```python
from build123d import *

# Parameters (mm, degrees)
F0_R          = 3
F0_R_2        = 2.5
F1_DEPTH      = 1100.6
F2_R          = 2
F3_R          = 7
F5_DEPTH      = 30
F5_DEPTH_BACK = 30


# Not quite as in the source:
# - a feature names something its author has since deleted; it is built from what else it names


with BuildPart() as f1:
    # F0 (on Top) → F1 (new body)
    with BuildSketch(Plane.XY):
        with BuildLine():
            Line((18.15, -30), (30, -30))
            Line((30, -30), (30, -18.15))
            Line((30, -18.15), (27.5, -18.15))
            Line((27.5, -18.15), (27.5, -20.15))
            Line((27.5, -20.15), (21.5477069044, -20.15))
            ThreePointArc((21.5477069044, -20.15), (19.5, -15), (21.5477069044, -9.85))
            Line((21.5477069044, -9.85), (27.5, -9.85))
            Line((27.5, -9.85), (27.5, -11.85))
            Line((27.5, -11.85), (30, -11.85))
            Line((30, -11.85), (30, 11.85))
            Line((30, 11.85), (27.5, 11.85))
            Line((27.5, 11.85), (27.5, 9.85))
            Line((27.5, 9.85), (21.5477069044, 9.85))
            ThreePointArc((21.5477069044, 9.85), (19.5, 15), (21.5477069044, 20.15))
            Line((21.5477069044, 20.15), (27.5, 20.15))
            Line((27.5, 20.15), (27.5, 18.15))
            Line((27.5, 18.15), (30, 18.15))
            Line((30, 18.15), (30, 30))
            Line((30, 30), (18.15, 30))
            Line((18.15, 30), (18.15, 27.5))
            Line((18.15, 27.5), (20.15, 27.5))
            Line((20.15, 27.5), (20.15, 21.5477069044))
            ThreePointArc((20.15, 21.5477069044), (15, 19.5), (9.85, 21.5477069044))
            Line((9.85, 21.5477069044), (9.85, 27.5))
            Line((9.85, 27.5), (11.85, 27.5))
            Line((11.85, 27.5), (11.85, 30))
            Line((11.85, 30), (-11.85, 30))
            Line((-11.85, 30), (-11.85, 27.5))
            Line((-11.85, 27.5), (-9.85, 27.5))
            Line((-9.85, 27.5), (-9.85, 21.5477069044))
            ThreePointArc((-9.85, 21.5477069044), (-15, 19.5), (-20.15, 21.5477069044))
            Line((-20.15, 21.5477069044), (-20.15, 27.5))
            Line((-20.15, 27.5), (-18.15, 27.5))
            Line((-18.15, 27.5), (-18.15, 30))
            Line((-18.15, 30), (-30, 30))
            Line((-30, 30), (-30, 18.15))
            Line((-30, 18.15), (-27.5, 18.15))
            Line((-27.5, 18.15), (-27.5, 20.15))
            Line((-27.5, 20.15), (-21.5477069044, 20.15))
            ThreePointArc((-21.5477069044, 20.15), (-19.5, 15), (-21.5477069044, 9.85))
            Line((-21.5477069044, 9.85), (-27.5, 9.85))
            Line((-27.5, 9.85), (-27.5, 11.85))
            Line((-27.5, 11.85), (-30, 11.85))
            Line((-30, 11.85), (-30, -11.85))
            Line((-30, -11.85), (-27.5, -11.85))
            Line((-27.5, -11.85), (-27.5, -9.85))
            Line((-27.5, -9.85), (-21.5477069044, -9.85))
            ThreePointArc((-21.5477069044, -9.85), (-19.5, -15), (-21.5477069044, -20.15))
            Line((-21.5477069044, -20.15), (-27.5, -20.15))
            Line((-27.5, -20.15), (-27.5, -18.15))
            Line((-27.5, -18.15), (-30, -18.15))
            Line((-30, -18.15), (-30, -30))
            Line((-30, -30), (-18.15, -30))
            Line((-18.15, -30), (-18.15, -27.5))
            Line((-18.15, -27.5), (-20.15, -27.5))
            Line((-20.15, -27.5), (-20.15, -21.5477069044))
            ThreePointArc((-20.15, -21.5477069044), (-15, -19.5), (-9.85, -21.5477069044))
            Line((-9.85, -21.5477069044), (-9.85, -27.5))
            Line((-9.85, -27.5), (-11.85, -27.5))
            Line((-11.85, -27.5), (-11.85, -30))
            Line((-11.85, -30), (11.85, -30))
            Line((11.85, -30), (11.85, -27.5))
            Line((11.85, -27.5), (9.85, -27.5))
            Line((9.85, -27.5), (9.85, -21.5477069044))
            ThreePointArc((9.85, -21.5477069044), (15, -19.5), (20.15, -21.5477069044))
            Line((20.15, -21.5477069044), (20.15, -27.5))
            Line((20.15, -27.5), (18.15, -27.5))
            Line((18.15, -27.5), (18.15, -30))
        make_face()
        with Locations((-25, -25)):
            Circle(F0_R, mode=Mode.SUBTRACT)
        with Locations((-15, -15)):
            Circle(F0_R_2, mode=Mode.SUBTRACT)
        with Locations((25, -25)):
            Circle(F0_R, mode=Mode.SUBTRACT)
        with Locations((15, -15)):
            Circle(F0_R_2, mode=Mode.SUBTRACT)
        with Locations((-25, 25)):
            Circle(F0_R, mode=Mode.SUBTRACT)
        with Locations((-15, 15)):
            Circle(F0_R_2, mode=Mode.SUBTRACT)
        Polygon((-7, 22), (-7, 27.5), (0, 27.5), (7, 27.5), (7, 22), (10, 16), (10, 10), (16, 10), (22, 7), (27.5, 7), (27.5, 0), (27.5, -7), (22, -7), (16, -10), (10, -10), (10, -16), (7, -22), (7, -27.5), (0, -27.5), (-7, -27.5), (-7, -22), (-10, -16), (-10, -10), (-16, -10), (-22, -7), (-27.5, -7), (-27.5, 0), (-27.5, 7), (-22, 7), (-16, 10), (-10, 10), (-10, 16), align=None, mode=Mode.SUBTRACT)
        with Locations((15, 15)):
            Circle(F0_R_2, mode=Mode.SUBTRACT)
        with Locations((25, 25)):
            Circle(F0_R, mode=Mode.SUBTRACT)
    extrude(amount=F1_DEPTH)

    # F2
    f2_edges = [f1.edges().sort_by_distance(p)[0] for p in [
        (-7, 27.5, 550.3),
        (7, 27.5, 550.3),
    ]]
    fillet(f2_edges, radius=F2_R)

    # F3
    f3_edges = [f1.edges().sort_by_distance(p)[0] for p in [
        (-10, 16, 550.3),
        (10, 16, 550.3),
    ]]
    fillet(f3_edges, radius=F3_R)

    # F4 (on Right) → F5 (cut, two sides)
    with BuildSketch(Plane.YZ) as f5_sk:
        Polygon((-164.2855995683, 38.6458085579), (-188.5911429791, -83.5464097089), (5.6944565892, -122.1922182668), (30, 0), align=None)
    extrude(amount=F5_DEPTH, mode=Mode.SUBTRACT)
    extrude(f5_sk.sketch, amount=-F5_DEPTH_BACK, mode=Mode.SUBTRACT)


solid = f1.part
```
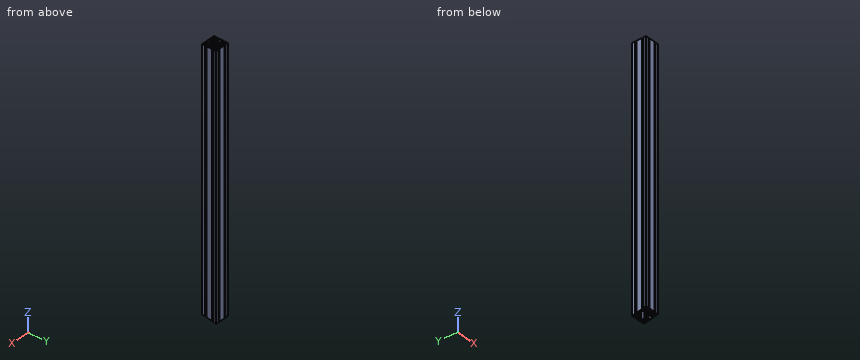
CAD build for the part. Positions are in the model's coordinates, mm. Round coordinates to 2 decimals unless told otherwise and drop trailing zeros. Return JSON: item names as keys, results as strings. Group by question number.
(1) Drop flat-ended pins along their axis: P1, Ø5, axis at x = 20, y = -15.5, coming from the -Z side; P2, Ø8, axis at x = 25, y = 25, coming from the -Z side; P3, Ø5, axis at x = 25, y = -25, coming from the -Z side (3 decimals); P4, Ø2, axis at x = 9.5, y = 12, coming from the -Z side. Give the stop position or say it passes through.
(2) Saw through at A-A, the plane z = 914. Give the number of separate pieces and of enclosed holes in the cut face, and give its area (3 significant figures).
(3) Wall check: probe 1 along Y at (x, z) = (-15, 679); probe 2 along X at (y, z) = (-25, 568); probe 3 along X at (y, z) = (-4, 291). Give the ranges that are in metal, low to high. Write a range as [from, to].
Answer list:
{
 "1": {"P1": "z = 8.56", "P2": "z = 0.2", "P3": "through", "P4": "z = 3.41"},
 "2": {"separate pieces": "1", "enclosed holes": "9", "area": "1,080 mm2"},
 "3": {"probe 1": "[-19.5, -17.5], [-12.5, -10], [10, 12.5], [17.5, 19.5]", "probe 2": "[-30, -28], [-22, -20.15], [-9.85, -7], [7, 9.85], [20.15, 22], [28, 30]", "probe 3": "[-30, -27.5], [27.5, 30]"}
}
